Can you work these out from the model? Positions are in its coordinate system, mm. Face numbers are marked on the shaded views. A direction names the side the tool comes from. Give positions to 0.01 mm unless a question says otherwise; leave off trailing zeros. Order: outer loops, then holes, each group sorted by start corner. A loop starts at its lowest first (then second) coordinate and runs counter-clockwise, first axis right, second up. Notation, with made-up numbers: (86, 84.25) - (145, 84.25) arc R22 cw to (145, 120.25) - close; hole circle Ø8 at (50, -17). An arc over 180 degrees is marked (long way). Return JSON: item names as keys, results as strings.
```python
from build123d import *

# Parameters (mm, degrees)
SKETCH1_R           = 15
BOSS_EXTRUDE1_DEPTH = 50
CUT_EXTRUDE1_DEPTH  = 20
CUT_EXTRUDE2_DEPTH  = 30


with BuildPart() as part:
    # Sketch1 → Boss-Extrude1 (new body)
    with BuildSketch(Plane(origin=(0, 0, 0), x_dir=(1, 0, 0), z_dir=(0, 1, 0))):
        Circle(SKETCH1_R)
    extrude(amount=BOSS_EXTRUDE1_DEPTH)

    # Sketch2 → Cut-Extrude1 (cut)
    with BuildSketch(Plane(origin=(0, 50, 0), x_dir=(1, 0, 0), z_dir=(0, 1, 0))):
        with BuildLine():
            Line((-3.709447398, 3.5), (3.709447398, 3.5))
            ThreePointArc((3.709447398, 3.5), (0, -5.1), (-3.709447398, 3.5))
        make_face()
    extrude(amount=-CUT_EXTRUDE1_DEPTH, mode=Mode.SUBTRACT)

    # Sketch3 → Cut-Extrude2 (cut)
    with BuildSketch(Plane.XZ):
        Polygon((-6.5, 0), (-3.25, 5.629165125), (3.25, 5.629165125), (6.5, 0), (3.25, -5.629165125), (-3.25, -5.629165125), align=None)
    extrude(amount=-CUT_EXTRUDE2_DEPTH, mode=Mode.SUBTRACT)


solid = part.part
```
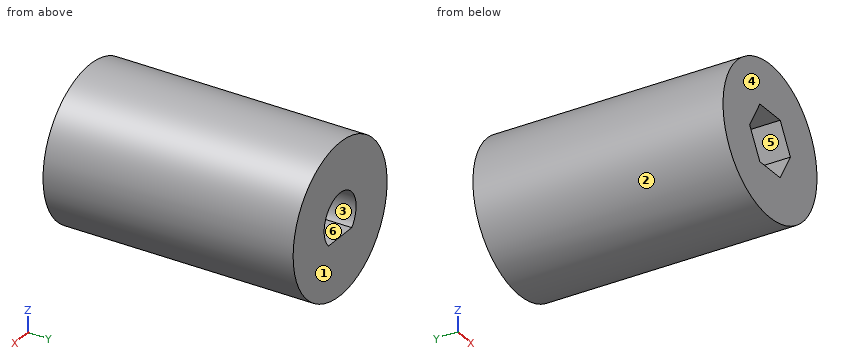
1. Suppose I cut it at A-A (x = 0). List the corners of the cut face in (y, z) for me, plus the area to 3 significant figures.
Checks:
{"outline": "(0, -15) - (50, -15) - (50, -3.5) - (30, -3.5) - (30, -5.63) - (0, -5.63) - close; (0, 5.63) - (30, 5.63) - (30, 5.1) - (50, 5.1) - (50, 15) - (0, 15) - close", "area": "990 mm^2"}
2. Suppose I cut it at D-D (z = -11). List the corners of the cut face in (x, y) for me.
Checks:
{"outline": "(-10.2, 0) - (10.2, 0) - (10.2, 50) - (-10.2, 50) - close"}
3. Suppose I cut it at B-B (y = 19.5). List the corners of the cut face in (x, z) for me, plus the area to 3 significant figures.
Checks:
{"outline": "circle Ø30 at (0, 0); hole (-6.5, 0) - (-3.25, -5.63) - (3.25, -5.63) - (6.5, 0) - (3.25, 5.63) - (-3.25, 5.63) - close", "area": "597 mm^2"}
4. If I drill on L1, parallel to Z at x = 0, y = 44.75; L2, parallel to X at y = 40.5, z = 0; L3, parallel to Z at x = 0.25, y = 6, over which ranges is the centre line in solid material (lowest first)? Write a range as [from, to].
Checks:
{"L1": "[-15, -3.5], [5.1, 15]", "L2": "[-15, -5.1], [5.1, 15]", "L3": "[-15, -5.63], [5.63, 15]"}
5. Thinking about a two-plate mould opening in X: for the marked faces 1, 2 and 3, which applies, +X half, -X half, draft (parallel to the pull), parting line (faces both ways), or undercut?
Checks:
{"face 1": "draft", "face 2": "parting line", "face 3": "undercut"}
6. On a 3-axis mill with a long thin cutter (end or side, diameter ignored), from which of +Z, -Z, +X, -X, +Y, -Y can I reach the whole of each face in a straight line? I mean the marked faces 4, 5 and 6. Say none if no direction works.
Checks:
{"face 4": "+Z, -Z, +X, -X, -Y", "face 5": "-Y", "face 6": "+Y, -Y"}
7. Suppose I cut it at C-C (x = -4.5). List the corners of the cut face in (y, z) for me, plus the area to 3 significant figures.
Checks:
{"outline": "(0, -14.31) - (50, -14.31) - (50, -2.4) - (30, -2.4) - (30, -3.46) - (0, -3.46) - close; (0, 3.46) - (30, 3.46) - (30, 2.4) - (50, 2.4) - (50, 14.31) - (0, 14.31) - close", "area": "1,130 mm^2"}
8. For pin 1 Ø6 at (x, z) = (0, 0) entering from -Y; pin 2 Ø5 at (y, z) = (42, 4) entering from +X; pin 3 Ø2 at (x, y) = (-10.5, 14.5) entering from +Z; pin 4 Ø1 at (x, y) = (-4, 25.5) entering from -Z, each with a flat end and sliding along its axis, tell me the tip position at first contact or that it passes through.
Checks:
{"pin 1": "through", "pin 2": "x = 14.92", "pin 3": "z = 11.61", "pin 4": "z = -14.59"}
